```python
from build123d import *

# Parameters (mm, degrees)
F0_R     = 4
F1_DEPTH = 45
F2_R     = 2


with BuildPart() as f1:
    # F0 (on Top) → F1 (new body, symmetric)
    with BuildSketch(Plane.XY):
        with BuildLine():
            ThreePointArc((-6.8818602136, -5.8), (3.0873336455, -8.4538967915), (9, 0))
            ThreePointArc((9, 0), (-0.5510337779, 8.9831153714), (-8.932524839, -1.1))
            ThreePointArc((-8.932524839, -1.1), (-8.2490116771, -3.5991396682), (-6.8818602136, -5.8))
        make_face()
        Circle(F0_R, mode=Mode.SUBTRACT)
        with BuildLine():
            ThreePointArc((-6.8818602136, -5.8), (-8.2490116771, -3.5991396682), (-8.932524839, -1.1))
            Line((-8.932524839, -1.1), (-17.7, -1.1))
            ThreePointArc((-17.7, -1.1), (-17.9121320344, -1.1878679656), (-18, -1.4))
            ThreePointArc((-18, -1.4), (-18.0878679656, -1.1878679656), (-18.3, -1.1))
            Line((-18.3, -1.1), (-19.8, -1.1))
            ThreePointArc((-19.8, -1.1), (-20.0121320344, -1.1878679656), (-20.1, -1.4))
            ThreePointArc((-20.1, -1.4), (-20.1878679656, -1.1878679656), (-20.4, -1.1))
            Line((-20.4, -1.1), (-21.7159694135, -1.1))
            Line((-21.7159694135, -1.1), (-21.9, -1.1))
            ThreePointArc((-21.9, -1.1), (-22.1121320344, -1.1878679656), (-22.2, -1.4))
            ThreePointArc((-22.2, -1.4), (-22.2878679656, -1.1878679656), (-22.5, -1.1))
            Line((-22.5, -1.1), (-25.77, -1.1))
            ThreePointArc((-25.77, -1.1), (-27.1842135624, -1.6857864376), (-27.77, -3.1))
            Line((-27.77, -3.1), (-27.77, -4.8))
            ThreePointArc((-27.77, -4.8), (-27.4771067812, -5.5071067812), (-26.77, -5.8))
            Line((-26.77, -5.8), (-24.35, -5.8))
            ThreePointArc((-24.35, -5.8), (-23.5721825407, -6.1221825407), (-23.25, -6.9))
            Line((-23.25, -6.9), (-23.25, -7.5))
            ThreePointArc((-23.25, -7.5), (-23.5721825407, -8.2778174593), (-24.35, -8.6))
            Line((-24.35, -8.6), (-25.05, -8.6))
            ThreePointArc((-25.05, -8.6), (-25.4035533906, -8.7464466094), (-25.55, -9.1))
            Line((-25.55, -9.1), (-25.55, -10.0435914154))
            ThreePointArc((-25.55, -10.0435914154), (-25.2571067812, -10.7506981966), (-24.55, -11.0435914154))
            Line((-24.55, -11.0435914154), (-21.4, -11.0435914154))
            ThreePointArc((-21.4, -11.0435914154), (-21.3121320344, -10.8314593811), (-21.1, -10.7435914154))
            Line((-21.1, -10.7435914154), (-20.4, -10.7435914154))
            ThreePointArc((-20.4, -10.7435914154), (-20.1878679656, -10.6557234498), (-20.1, -10.4435914154))
            ThreePointArc((-20.1, -10.4435914154), (-20.0121320344, -10.6557234498), (-19.8, -10.7435914154))
            Line((-19.8, -10.7435914154), (-19.1, -10.7435914154))
            ThreePointArc((-19.1, -10.7435914154), (-18.8878679656, -10.8314593811), (-18.8, -11.0435914154))
            Line((-18.8, -11.0435914154), (-15.65, -11.0435914154))
            ThreePointArc((-15.65, -11.0435914154), (-14.9428932188, -10.7506981966), (-14.65, -10.0435914154))
            Line((-14.65, -10.0435914154), (-14.65, -9.1))
            ThreePointArc((-14.65, -9.1), (-14.7964466094, -8.7464466094), (-15.15, -8.6))
            Line((-15.15, -8.6), (-15.85, -8.6))
            ThreePointArc((-15.85, -8.6), (-16.6278174593, -8.2778174593), (-16.95, -7.5))
            Line((-16.95, -7.5), (-16.95, -6.9))
            ThreePointArc((-16.95, -6.9), (-16.6278174593, -6.1221825407), (-15.85, -5.8))
            Line((-15.85, -5.8), (-6.8818602136, -5.8))
        make_face()
    extrude(amount=F1_DEPTH, both=True)

    # F2
    f2_edges = [f1.edges().sort_by_distance(p)[0] for p in [
        (-6.88186, -5.8, 0),
        (-8.932525, -1.1, 0),
    ]]
    fillet(f2_edges, radius=F2_R)


solid = f1.part
```
Verification items for the finished model (mm, model axes). A direction names the side the tool comes from. Coordinates: 2 decimals unless noted, no trailing zeros. Write each loop counter-clockwise with the first axis right and the second up, starting at its lowest first coordinate (ties: lowest second). Pieces come first, ordered by that corner, then holes. Notation, with made-up numbers: M 47.5,-9 L 96.5,-9 A24 cw 96.5,9 Z; hole C 54,-12.75 d7. An arc over 180 degrees is marked long. Answer as a JSON object with one key per item and string values. Group by question number.
(1) Cross-section at B-B, the plane y = -2.25. Record the cut outline in (x, z), and give its area (3 significant figures).
(2) Material ranges on line 1 (Y direction, x = 0, z = 25); line 2 (Y direction, x = -14, z = 30); line 3 (X direction, y = -9.75, z = 14.5), recorded low to high.
(3) Cross-section at A-A, the plane x = -1.5. Record the cut outline in (y, z).
(4) Tool access check on faces 1 (the face through (-6, -1, -45)), 2 (the face through (-24, -1.1, 1)), 3 (the face through (-26, -5.8, 1)). Record the directions out of +Z, -Z, +X, -X, +Y, -Y that give a thin tool (end or side, any length) a straight path to the whole face; none if there is none.
(5) Gauge pin test, flat ends, axial feed: pin 1 (5 mm diameter, centred on y = 5.5, z = 26.5, fed in from -X); pin 2 (8 mm diameter, centred on x = -4.5, z = 23.5, fed in from -Y); pin 3 (1 mm diameter, centred on x = -24, z = 19.5, fed in from +Y). Record the tip position at first contact, or that the pin passes through.
(6) Release check for a two-part mould opening along X. For faces 4 (the face through (-14, -1.1, 1)), 5 (the face through (-27.77, -4, 1)), 6 (the face through (-0.867, -3.905, -0.63)) record: +X half, -X half, draft (parallel to the pull), parting line (faces both ways), or undercut.
Reply:
{
 "1": {"outline": "M -27.58,-45 L -3.31,-45 L -3.31,45 L -27.58,45 Z; M 3.31,-45 L 8.71,-45 L 8.71,45 L 3.31,45 Z", "area": "2,670 mm²"},
 "2": {"line 1": "-9 to -4, 4 to 9", "line 2": "-5.8 to -1.1", "line 3": "-25.55 to -14.65"},
 "3": {"outline": "M -8.87,-45 L -3.71,-45 L -3.71,45 L -8.87,45 Z; M 3.71,-45 L 8.87,-45 L 8.87,45 L 3.71,45 Z"},
 "4": {"face 1": "-Z, +X, -X, +Y, -Y", "face 2": "+Z, -Z, -X, +Y", "face 3": "+Z, -Z, -X"},
 "5": {"pin 1": "x = -8.49", "pin 2": "y = -8.99", "pin 3": "y = -1.1"},
 "6": {"face 4": "draft", "face 5": "-X half", "face 6": "undercut"}
}
